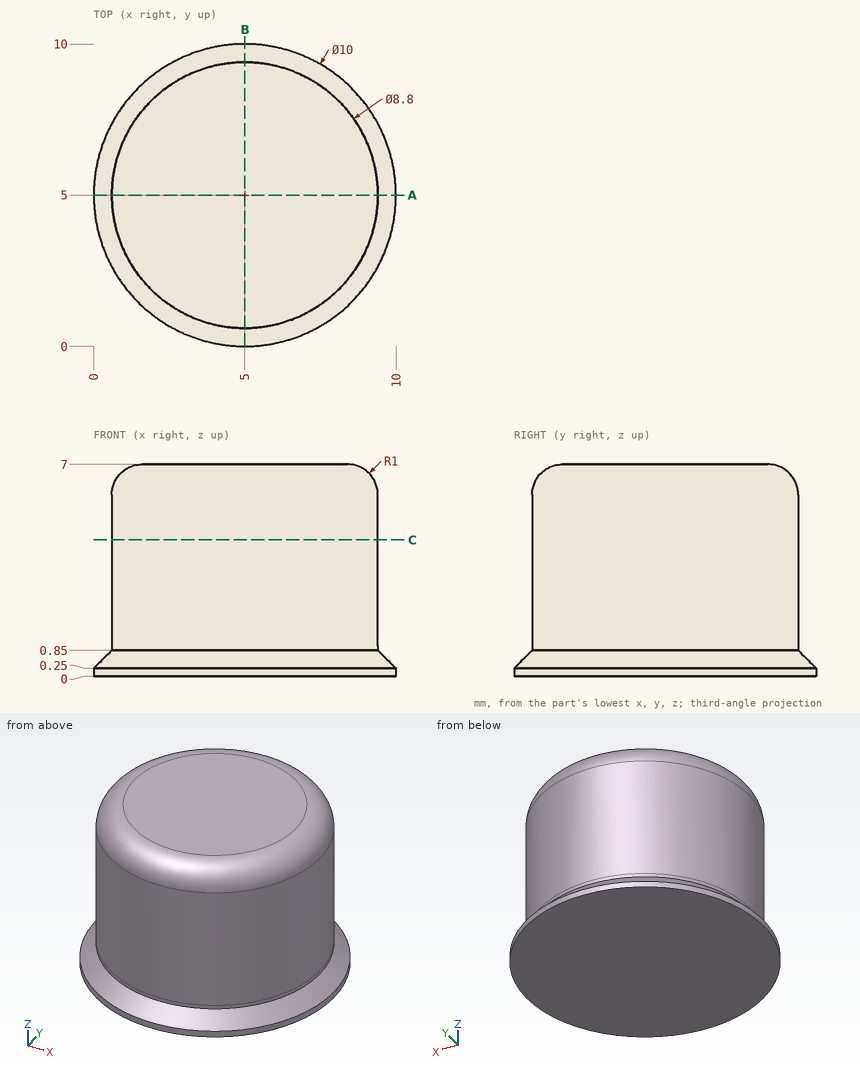
Can you work these out from the drawing? Everything is in mm from the part's minimum corner. Give positions to 0.01 mm unless a question says otherwise; leave off trailing zeros. Order: outer loops, then holes, each group sorted by start corner. A loop starts at its lowest first (then second) coordinate and runs counter-clockwise, first axis right, second up. Notation, with made-up numbers: M 82.5,52 L 109.5,52 A15 ccw 109.5,69 Z; hole C 46,38.5 d9. An arc over 180 degrees is marked long. Use a Markdown table: item, result. Add a question column.
1. Suppose I cut it at C-C (z = 4.5). List the corners of the cut face in (x, y) for me, and give its area (3 significant figures).
2. Suppose I cut it at A-A (y = 5). List the corners of the cut face in (x, z) for me.
3. I need wall thicknesses on probe 1 along Y at (x, z) = (7.75, 4); probe 2 along Z at (x, y) = (8, 2.75); probe 3 along Z at (x, y) = (8.5, 5). Which ranges of each line are inside material? Lowest first, please. Write a range as from..to.
4. For pin 1 Ø4 at (y, z) = (9, 4) entering from +X; pin 2 Ø4 at (x, z) = (4, 3.5) entering from -Y; pin 3 Ø3 at (x, z) = (7, 5.5) entering from +Y, each with a flat end and sliding along its axis, tell me the tip position at first contact or that it passes through.
Results list:
| question | item | result |
|---|---|---|
| 1 | outline | C 5,5 d8.8 |
| 1 | area | 60.8 mm² |
| 2 | outline | M 0,0 L 10,0 L 10,0.25 L 9.4,0.85 L 9.4,6 A1 ccw 8.4,7 L 1.6,7 A1 ccw 0.6,6 L 0.6,0.85 L 0,0.25 Z |
| 3 | probe 1 | y = 1.57..8.43 |
| 3 | probe 2 | z = 0..6.94 |
| 3 | probe 3 | z = 0..6.99 |
| 4 | pin 1 | stops at x = 8.92 |
| 4 | pin 2 | stops at y = 0.6 |
| 4 | pin 3 | stops at y = 9.37 |
